Input: part model. Units: mm. Frame: model coordinates. A direction names the side the tool comes from. Coordinates: 2 decimals unless noted, no trailing zeros. Write each loop counter-clockwise with the first axis right and the second up, starting at its lowest first coordinate (ties: lowest second). Pieces come first, ordered by that corner, then holes. Notation, with made-up numbers: (-34.5, 55.5) - (-28.5, 55.5) arc R16 ccw to (-28.5, 74.5) - close; hole circle Ø5 at (-23, -35.5). An arc over 180 degrees is marked (long way). Put each result on its own line as item: value. Start each with the question number.
1. Access query for faces 4 (the cylindrical face through (-56.797, 0.892, 6.014)), 5 (the cylindrical face through (46.73, 0.43, 0.73)). Directions: +Z, -Z, +X, -X, +Y, -Y. A direction counts if a zero-diameter tool reaches every point of the face in a straight line with its end or side. Return the directions, or none.
2. Pull-direction query (Y, two-part tool) for faces 1 (the flat face through (-1, -7.5, 3)), 2 (the conical face through (47.03, -1.894, 1.667)), 3 (the flat face through (-1, 0, 0)); classes: released by +Y, released by -Y, zero draft, split by the parting line, or undercut.
3. Line query: line 1 (X direction, y = 0, z = 1.15); line 2 (Y direction, x = 50, z = 6.25) (3 decimals); line 3 (X direction, y = -1.25, z = 5.25). Output: solid intervals per line, ascending.
4. Pin query (flat end, axial travel): pin 1 (8.5 mm diameter, centred on x = 50, y = 0, fed in from +Z) (3 decimals). Return the tip coordinate at first contact, or that it passes through.
5. Cut plane B-B, the plane y = 0. Return loops of the section in (x, z) (3 decimals), and give its area (3 significant figures).
6. Cut plane A-A, the plane x = -50. Return loops of the section in (y, z) (3 decimals), and give its area (3 significant figures).
from build123d import *

# Parameters (mm, degrees)
SKETCH_1_W                 = 200
SKETCH_1_H                 = 15
EXTRUDE_1_DEPTH            = 7
CHAMFER_1_SIZE             = 5
HOLE_WIZARD_M61_AT_2_COUNT = 2
HOLE_WIZARD_M61_AT_2_PITCH = 100


with BuildPart() as part:
    # Эскиз1 → Бобышка-Вытянуть1 (new body)
    with BuildSketch(Plane.XY):
        Rectangle(SKETCH_1_W, SKETCH_1_H)
    extrude(amount=EXTRUDE_1_DEPTH)

    # Фаска1
    chamfer_1_edges = [part.edges().sort_by_distance(p)[0] for p in [
        (100, 0, 7),
    ]]
    chamfer(chamfer_1_edges, length=CHAMFER_1_SIZE)

    # Эскиз4 → Зенковка для винта с потайной головкой и внутренним шестигранником M61 (revolve, cut)
    with BuildSketch(Plane(origin=(-50, 0, 7), x_dir=(0, -1, 0), z_dir=(1, 0, 0))):
        Polygon((0, 0), (0, 31.982840043), (3.3, 30), (3.3, 5.555), (6.855, 2), (6.855, 0), align=None)
    hole_wizard_m61 = revolve(axis=Axis((-50, 0, 13.35), (0, 0, -1)), mode=Mode.SUBTRACT)

    # Зенковка для винта с потайной головкой и внутренним шестигранником M61 at 2: Зенковка для винта с потайной головкой и внутренним шестигранником M61 ×2
    with Locations(*[(i * HOLE_WIZARD_M61_AT_2_PITCH, 0, 0) for i in range(1, HOLE_WIZARD_M61_AT_2_COUNT)]):
        add(hole_wizard_m61, mode=Mode.SUBTRACT)


solid = part.part
Report:
1. face 4: +Z
1. face 5: +Z, -Z
2. face 1: released by -Y
2. face 2: undercut
2. face 3: zero draft
3. line 1: x = -100 to -53.3, -46.7 to 46.7, 53.3 to 100
3. line 2: y = -7.5 to -6.855, 6.855 to 7.5
3. line 3: x = -100 to -56.74, -43.26 to 43.26, 56.74 to 96.75
4. pin 1: stops at z = 2.395
5. outline: (-100, 0) - (-53.3, 0) - (-53.3, 1.445) - (-56.855, 5) - (-56.855, 7) - (-100, 7) - close; (-46.7, 0) - (46.7, 0) - (46.7, 1.445) - (43.145, 5) - (43.145, 7) - (-43.145, 7) - (-43.145, 5) - (-46.7, 1.445) - close; (53.3, 0) - (100, 0) - (100, 2) - (95, 7) - (56.855, 7) - (56.855, 5) - (53.3, 1.445) - close
5. area: 1,240 mm^2
6. outline: (-7.5, 0) - (-3.3, 0) - (-3.3, 1.445) - (-6.855, 5) - (-6.855, 7) - (-7.5, 7) - close; (3.3, 0) - (7.5, 0) - (7.5, 7) - (6.855, 7) - (6.855, 5) - (3.3, 1.445) - close
6. area: 31.9 mm^2
